from build123d import *

# Parameters (mm, degrees)
PAD_DEPTH    = 2
PAD001_DEPTH = 7
PAD002_DEPTH = 14
ARRAY_COUNT  = 3


with BuildPart() as pad:
    # Sketch → Pad (new body)
    with BuildSketch(Plane.XY):
        Polygon((0, 0), (-7.7942286341, 13.5), (-68, 13.5), (-68, -13.5), (-7.7942286341, -13.5), align=None)
    extrude(amount=PAD_DEPTH)


with BuildPart() as pad001:
    # Sketch001 → Pad001 (new body)
    with BuildSketch(Plane.XY.offset(0.1)):
        Polygon((0, 0), (-1.443375673, 2.5), (-10, 2.5), (-10, 5), (-60, 5), (-60, -5), (-10, -5), (-10, -2.5), (-1.443375673, -2.5), align=None)
    extrude(amount=PAD001_DEPTH)


with BuildPart() as array:
    # Sketch002 → Pad002 (new body)
    with BuildSketch(Plane.XY):
        Polygon((-6.6395280957, 11.5), (-7.7942286341, 13.5), (-68, 13.5), (-68, -13.5), (-7.7942286341, -13.5), (-6.6395280957, -11.5), (-66, -11.5), (-66, 11.5), align=None)
    extrude(amount=PAD002_DEPTH)

    # Fusion: union Pad, Pad001
    add(pad.part)
    add(pad001.part)

    # Array: Array ×3 about axis
    array_axis = Axis((0, 0, 0), (0, 0, 1))


with BuildPart() as array_1:
    add(array.part)
    for i in range(1, ARRAY_COUNT):
        add(array.part.rotate(array_axis, i * 360 / ARRAY_COUNT))


solid = array_1.part
For this review, take the finished solid that the model builds, in its own axes (mm). A direction names the side the tool comes from. Round coordinates to 2 decimals unless told otherwise and drop trailing zeros. Order: outer loops, then holes, each group sorted by start corner. A loop starts at its lowest first (then second) coordinate and runs counter-clockwise, first axis right, second up. Notation, with made-up numbers: (55, 9) -> (108, 9) arc R34 ccw to (108, 41) -> close; hole circle Ø11 at (49, 43.5). An arc over 180 degrees is marked (long way). Write item = value, one per line. Start each with the question number.
1) Take a section at D-D on y = 47.5. State the section outline as (x, z) points, plus the area to 3 significant figures.
2) Take a section at A-A on z = 10.5. State the section outline as (x, y) points.
3) Take a section at C-C on x = 19. State the section outline as (y, z) points.
4) Tool access review of faces 4 (the face through (-38, -13.5, 7)), 5 (the face through (-37, 13.5, 7)), 6 (the face through (33.1, -57.1, 7.9)), 7 (the face through (30.85, -26.43, 6.9)): name each direction out of +Z, -Z, +X, -X, +Y, -Y from which nothing blocks a thin tool from reaching the whole face with its end or side.
5) Take a section at B-B on x = -48. State the section outline as (y, z) points, plus the area to 3 significant figures.
6) To check wall thickness, follow line 1 (Y direction, x = -54, z = 3.5); line 2 (Y direction, x = 14.5, z = 4.25); line 3 (Y direction, x = -36, z = 11.75). State the ranges of each line that lie inside material, in increasing order. Write a range as from..to.
7) The part is to be moulded in two halves that separate along Y. For faces 1 (the face through (34.164, 58.795, 6.902)), 2 (the face through (33.84, -58.98, 6.9)), 3 (the face through (21.655, 27.508, 4.514)), say which applies: +Y half, -Y half, draft (parallel to the pull), parting line (faces both ways), or undercut.
8) Insertion check: pin 1 (7 mm diameter, centred on x = -49.5, z = 5, fed in from -Y); pin 2 (2 mm diameter, centred on y = -21.5, z = 11, fed in from +X); pin 3 (5.5 mm diameter, centred on x = -6, z = 3.5, fed in from -Y). Each pin has a flat end and moves straight along its axis. Give the tip position at first contact, or say it passes through.
Verdict:
q1.outline = (11.84, 0) -> (43.01, 0) -> (43.01, 14) -> (40.7, 14) -> (40.7, 2) -> (33.2, 2) -> (33.2, 7.1) -> (21.65, 7.1) -> (21.65, 2) -> (14.15, 2) -> (14.15, 14) -> (11.84, 14) -> close
q1.area = 177 mm2
q2.outline = (-68, -13.5) -> (-7.79, -13.5) -> (22.31, -65.64) -> (45.69, -52.14) -> (15.59, 0) -> (45.69, 52.14) -> (22.31, 65.64) -> (-7.79, 13.5) -> (-68, 13.5) -> close; hole (-66, -11.5) -> (-6.64, -11.5) -> (23.04, -62.91) -> (42.96, -51.41) -> (13.28, 0) -> (42.96, 51.41) -> (23.04, 62.91) -> (-6.64, 11.5) -> (-66, 11.5) -> close
q3.outline = (-59.91, 0) -> (-5.91, 0) -> (-5.91, 14) -> (-9.91, 14) -> (-9.91, 2) -> (-22.91, 2) -> (-22.91, 7.1) -> (-42.91, 7.1) -> (-42.91, 2) -> (-55.91, 2) -> (-55.91, 14) -> (-59.91, 14) -> close; (5.91, 0) -> (59.91, 0) -> (59.91, 14) -> (55.91, 14) -> (55.91, 2) -> (42.91, 2) -> (42.91, 7.1) -> (22.91, 7.1) -> (22.91, 2) -> (9.91, 2) -> (9.91, 14) -> (5.91, 14) -> close
q4.face_4 = +Z, -Z, -X, -Y
q4.face_5 = +Z, -Z, -X, +Y
q4.face_6 = +Z
q4.face_7 = +Z, -Z, +X
q5.outline = (-13.5, 0) -> (13.5, 0) -> (13.5, 14) -> (11.5, 14) -> (11.5, 2) -> (5, 2) -> (5, 7.1) -> (-5, 7.1) -> (-5, 2) -> (-11.5, 2) -> (-11.5, 14) -> (-13.5, 14) -> close
q5.area = 153 mm2
q6.line_1 = -13.5..-11.5, -5..5, 11.5..13.5
q6.line_2 = -52.11..-48.11, -35.11..-15.11, -2.11..2.11, 15.11..35.11, 48.11..52.11
q6.line_3 = -13.5..-11.5, 11.5..13.5
q7.face_1 = +Y half
q7.face_2 = -Y half
q7.face_3 = undercut
q8.pin_1 = -13.5
q8.pin_2 = 28.58
q8.pin_3 = -21.37
